For this review, take the finished solid that the model builds, in its own axes (mm). Give positions to 0.01 mm unless a question says otherwise; leave off trailing zeros. Loops run counter-clockwise (first coordinate to the right, second up) from the corner with the lowest first, then second, coordinate; pieces in that order, holes last.
```python
from build123d import *

# Parameters (mm, degrees)
REVOLVE1_ANGLE     = 180
SKETCH2_R          = 44.45
CUT_EXTRUDE1_DEPTH = 2
F_30DEG_W          = 1
F_30DEG_H          = 1


with BuildPart() as part:
    # Sketch1 → Revolve1 (revolve)
    with BuildSketch(Plane(origin=(0, 0, 0), x_dir=(1, 0, 0), z_dir=(0, 1, 0))):
        with BuildLine():
            ThreePointArc((0, 44.45), (-44.45, 0), (0, -44.45))
            Line((0, -44.45), (0, -42.45))
            ThreePointArc((0, -42.45), (-42.45, 0), (0, 42.45))
            Line((0, 42.45), (0, 44.45))
        make_face()
    revolve(axis=Axis((0, 0, 44.45), (0, 0, -1)), revolution_arc=REVOLVE1_ANGLE)

    # Sketch2 → Cut-Extrude1 (cut)
    with BuildSketch(Plane(origin=(0, 0, 0), x_dir=(1, 0, 0), z_dir=(0, 1, 0))):
        Circle(SKETCH2_R)
    extrude(amount=CUT_EXTRUDE1_DEPTH, mode=Mode.SUBTRACT)

    # 30deg → Cut-Revolve1 (revolve, cut)
    with BuildSketch(Plane(origin=(0, 0, 0), x_dir=(0, 0, -1), z_dir=(1, 0, 0))):
        with Locations((43.95, 0)):
            Rectangle(F_30DEG_W, F_30DEG_H)
        Polygon((38.244829198, 22.658012702), (38.744829198, 21.791987298), (37.878803794, 21.291987298), (37.378803794, 22.158012702), align=None)
        Polygon((21.791987298, 38.744829198), (22.658012702, 38.244829198), (22.158012702, 37.378803794), (21.291987298, 37.878803794), align=None)
    revolve(axis=Axis((0, -1000, 0), (0, 1, 0)), mode=Mode.SUBTRACT)


solid = part.part
```
Item 1: Take a section at C-C on y = 34.5. Give the boundary of the cut face in (x, z).
Answer:
outline: circle Ø56.06 at (0, 0); hole circle Ø49.47 at (0, 0)
Item 2: For L1, parallel to X at y = 7.5, z = -8; L2, parallel to Z at x = 11, y = 37; L3, parallel to X at y = 4, z = -7, list the stretches that pass through material, from the lowest coordinate up.
Answer:
L1: x = -43.08 to -41.01, 41.01 to 43.08
L2: z = -22.04 to -17.66, 17.66 to 22.04
L3: x = -43.71 to -41.68, 41.68 to 43.71
Item 3: Clearance check with flat-ended pins moving along their axes: pin 1 Ø1 at (x, y) = (10.5, 17) entering from +Z; pin 2 Ø10 at (y, z) = (30.5, -20.5) entering from -X; pin 3 Ø6 at (y, z) = (20, 34.5) entering from -X; pin 4 Ø10 at (x, z) = (35, -13.5) entering from -Y. State where each tip first meets the part, or that it passes through.
Answer:
pin 1: stops at z = 39.95
pin 2: stops at x = -31.11
pin 3: stops at x = -24.82
pin 4: stops at y = 2
